from build123d import *

# Parameters (mm, degrees)
F1_W     = 42.3
F1_H     = 42.3
F1_R     = 1.625
F2_DEPTH = 50
F4_T     = -3
F5_D     = 3.4
F6_D     = 6.6
F7_D     = 22.5
F8_SIZE  = 40
F9_R     = 3


with BuildPart() as f2:
    # F1 (on Top) → F2 (new body)
    with BuildSketch(Plane.XY):
        Rectangle(F1_W, F1_H)
        with Locations((-15.5, -15.5)):
            Circle(F1_R, mode=Mode.SUBTRACT)
        with Locations((15.5, -15.5)):
            Circle(F1_R, mode=Mode.SUBTRACT)
        with Locations((-15.5, 15.5)):
            Circle(F1_R, mode=Mode.SUBTRACT)
        with Locations((15.5, 15.5)):
            Circle(F1_R, mode=Mode.SUBTRACT)
        with Locations((-15.5, 15.5)):
            Circle(F1_R)
        with Locations((15.5, 15.5)):
            Circle(F1_R)
        with Locations((-15.5, -15.5)):
            Circle(F1_R)
        with Locations((15.5, -15.5)):
            Circle(F1_R)
        Polygon((-21.15, 21.15), (21.15, 21.15), (21.15, -21.15), (24.15, -21.15), (24.15, 24.15), (-24.15, 24.15), (-24.15, -21.15), (-21.15, -21.15), align=None)
    extrude(amount=F2_DEPTH)

    # F4
    f4_openings = [f2.faces().sort_by_distance(p)[0] for p in [
        (0, -21.15, 25),
        (0, 1.5, 0),
    ]]
    offset(amount=F4_T, openings=f4_openings)

    # F5 (through all)
    with Locations(Plane(origin=(0, 0, 0), x_dir=(1, 0, 0), z_dir=(0, 0, -1))):
        with Locations((-15.5, 15.5), (15.5, 15.5), (15.5, -15.5), (-15.5, -15.5)):
            Hole(F5_D / 2)

    # F6 (through all)
    with Locations(Plane.XZ.offset(21.15)):
        with Locations((0, 33.5), (0, 13.5)):
            Hole(F6_D / 2)

    # F7 (through all)
    with Locations(Plane(origin=(0, 0, 0), x_dir=(1, 0, 0), z_dir=(0, 0, -1))):
        with Locations((0, 0)):
            Hole(F7_D / 2)

    # F8
    f8_edges = [f2.edges().sort_by_distance(p)[0] for p in [
        (-22.65, -21.15, 0),
        (22.65, -21.15, 0),
    ]]
    chamfer(f8_edges, length=F8_SIZE)

    # F9 (call 1 of 8: OpenCascade refuses the feature's edges together)
    f9_edges = [f2.edges().sort_by_distance(p)[0] for p in [
        (-22.65, -21.15, 40),
    ]]
    fillet(f9_edges, radius=F9_R)

    # F9#2 (call 2 of 8)
    f9_2_edges = [f2.edges().sort_by_distance(p)[0] for p in [
        (22.65, -21.15, 40),
    ]]
    fillet(f9_2_edges, radius=F9_R)

    # F9#3 (call 3 of 8)
    f9_3_edges = [f2.edges().sort_by_distance(p)[0] for p in [
        (-22.65, 18.85, 0),
    ]]
    fillet(f9_3_edges, radius=F9_R)

    # F9#4 (call 4 of 8)
    f9_4_edges = [f2.edges().sort_by_distance(p)[0] for p in [
        (22.65, 18.85, 0),
    ]]
    fillet(f9_4_edges, radius=F9_R)

    # F9#5 (call 5 of 8)
    f9_5_edges = [f2.edges().sort_by_distance(p)[0] for p in [
        (-21.15, 21.15, 23.5),
    ]]
    fillet(f9_5_edges, radius=F9_R)

    # F9#6 (call 6 of 8)
    f9_6_edges = [f2.edges().sort_by_distance(p)[0] for p in [
        (21.15, 21.15, 23.5),
    ]]
    fillet(f9_6_edges, radius=F9_R)

    # F9#7 (call 7 of 8)
    f9_7_edges = [f2.edges().sort_by_distance(p)[0] for p in [
        (-24.15, 24.15, 25),
    ]]
    fillet(f9_7_edges, radius=F9_R)

    # F9#8 (call 8 of 8)
    f9_8_edges = [f2.edges().sort_by_distance(p)[0] for p in [
        (24.15, 24.15, 25),
    ]]
    fillet(f9_8_edges, radius=F9_R)


solid = f2.part
The model under review builds one solid part; all positions refer to its coordinate system, in mm. A direction names the side the tool comes from. Round coordinates to 2 decimals unless told otherwise and drop trailing zeros. Order: outer loops, then holes, each group sorted by start corner. A loop starts at its lowest first (then second) coordinate and runs counter-clockwise, first axis right, second up. Notation, with made-up numbers: (50, 61.5) -> (54, 61.5) arc R19 cw to (54, 95.5) -> close; hole circle Ø11 at (-3.75, 71.25). An arc over 180 degrees is marked (long way). Return JSON: item names as keys, results as strings.
1. For faces 1 (the face through (22.73, 18.96, 0.22)), 2 (the face through (9, -9, 47)), list the 3-axis set-ups (+Z, -Z, +X, -X, +Y, -Y) from which the entire face can be reached by the end or side of a thin tool; tool diameter is ignored.
Answer block:
{"face 1": "-Z, +X, -X, -Y", "face 2": "-Z, -Y"}
2. For L1, parallel to Y at x = 15.5, z = 47.6; L2, parallel to X at y = -15.5, z = 47.95; L3, parallel to X at y = -6, z = 32, list the stretches that pass through material, from the lowest coordinate up. Write a range as [from, to].
Answer block:
{"L1": "y = [-21.15, -17.2], [-13.8, 13.8], [17.2, 24.15]", "L2": "x = [-24.15, -17.2], [-13.8, 13.8], [17.2, 24.15]", "L3": "x = [-24.15, -21.15], [21.15, 24.15]"}
3. Take a section at D-D (y = -15.5). Write out the cut boundary in (x, z), then the cut area to 3 significant figures.
Answer block:
{"outline": "(-24.15, 34.35) -> (-21.15, 34.35) -> (-21.15, 47) -> (-17.2, 47) -> (-17.2, 50) -> (-24.15, 50) -> close; (-13.8, 47) -> (13.8, 47) -> (13.8, 50) -> (-13.8, 50) -> close; (17.2, 47) -> (21.15, 47) -> (21.15, 34.35) -> (24.15, 34.35) -> (24.15, 50) -> (17.2, 50) -> close", "area": "200 mm²"}
4. The part is to be moulded in two halves that separate along Z. For faces 3 (the face through (0, 12, 50)), 4 (the face through (-1.774, 22.671, 36.283)), 5 (the face through (-21.15, 3, 29)), say which applies: +Z half, -Z half, draft (parallel to the pull), parting line (faces both ways), or undercut.
Answer block:
{"face 3": "+Z half", "face 4": "undercut", "face 5": "draft"}
5. Take a section at B-B (z = 13.5). Write out the cut boundary in (x, y), then the cut area to 3 significant figures.
Answer block:
{"outline": "(-24.15, 5.35) -> (-21.15, 5.35) -> (-21.15, 18.15) arc R3 cw to (-18.15, 21.15) -> (-3.3, 21.15) -> (-3.3, 24.15) -> (-21.15, 24.15) arc R3 ccw to (-24.15, 21.15) -> close; (3.3, 21.15) -> (18.15, 21.15) arc R3 cw to (21.15, 18.15) -> (21.15, 5.35) -> (24.15, 5.35) -> (24.15, 21.15) arc R3 ccw to (21.15, 24.15) -> (3.3, 24.15) -> close", "area": "220 mm²"}
6. Take a section at A-A (x = 0). Write out the cut boundary in (y, z).
Answer block:
{"outline": "(-21.15, 47) -> (-11.25, 47) -> (-11.25, 50) -> (-21.15, 50) -> close; (11.25, 47) -> (21.15, 47) -> (21.15, 36.8) -> (24.15, 36.8) -> (24.15, 50) -> (11.25, 50) -> close; (21.15, 0) -> (24.15, 0) -> (24.15, 10.2) -> (21.15, 10.2) -> close; (21.15, 16.8) -> (24.15, 16.8) -> (24.15, 30.2) -> (21.15, 30.2) -> close"}
7. Insertion check: P1, Ø10, axis at x = 10, y = 11, coming from the -Z side; P2, Ø11, axis at x = -2, z = 26, coming from the -Y side. Each pin has a flat end and moves straight along its axis. Give the tip position at first contact, or say it passes through.
Answer block:
{"P1": "stops at z = 47", "P2": "stops at y = 21.15"}
8. Take a section at C-C (x = 15.5). Write out the cut boundary in (y, z), then the cut area to 4 significant figures.
Answer block:
{"outline": "(-21.15, 47) -> (-17.2, 47) -> (-17.2, 50) -> (-21.15, 50) -> close; (-13.8, 47) -> (13.8, 47) -> (13.8, 50) -> (-13.8, 50) -> close; (17.2, 47) -> (21.15, 47) -> (21.15, 0) -> (24.15, 0) -> (24.15, 50) -> (17.2, 50) -> close", "area": "256.5 mm²"}
